from build123d import *

# Parameters (mm, degrees)
F0_W          = 44.958
F0_H          = 48.133
F1_DEPTH      = 0.8001
F2_R          = 5.207
F3_DEPTH      = 25.4
F3_DEPTH_BACK = 6.35
F4_W          = 12.7
F4_H          = 35.433
F5_DEPTH      = 19.05


with BuildPart() as f1:
    # F0 (on Top) → F1 (new body, symmetric)
    with BuildSketch(Plane.XY):
        Rectangle(F0_W, F0_H)
    extrude(amount=F1_DEPTH, both=True)



with BuildPart() as f3:
    # F2 (on face) → F3 (new body, two sides)
    with BuildSketch(Plane.XZ.offset(24.0665)) as f3_sk:
        with Locations((11.684, 11.5189)):
            Circle(F2_R)
    extrude(amount=F3_DEPTH)
    extrude(f3_sk.sketch, amount=-F3_DEPTH_BACK)


with BuildPart() as f1_1:
    add(f1.part)

    add(f3.part)  # F5 merges F3
    # F4 (on face) → F5 (join)
    with BuildSketch(Plane.XY.offset(0.8001)):
        with Locations((11.684, 0)):
            Rectangle(F4_W, F4_H)
    extrude(amount=F5_DEPTH)


solid = f1_1.part
Can you work these out from the model? Positions are in its coordinate system, mm. A direction names the side the tool comes from. Coordinates: 2 decimals unless noted, no trailing zeros. Loops run counter-clockwise (first coordinate to the right, second up) from the corner with the lowest first, then second, coordinate; pieces in that order, holes last. Notation, with made-up numbers: M 33,-5 L 74,-5 A17 cw 74,4 Z; hole C 61,58.25 d3. An arc over 180 degrees is marked long. Return JSON: item names as keys, results as strings. Group by question number.
Item 1: On a 3-axis mill with a long thin cutter (end or side, diameter ignored), from which of +Z, -Z, +X, -X, +Y, -Y can I reach the whole of each face in a straight line? I mean faces 1 (the flat face through (0, -24.066, 0)), 2 (the flat face through (18.034, 0, 10)), 3 (the flat face through (12, -17.716, 6)), 4 (the flat face through (12, 17.716, 10)). Say none if no direction works.
Item 2: Imagine slicing it at A-A (y = -16). Please give me the cut outline in (x, z), and give its area (3 significant figures).
Item 3: I'm going to push flat-ended pins straight in: pin 1 Ø5 at (x, z) = (12.5, 1.5) entering from +Y; pin 2 Ø1.5 at (y, z) = (-15.5, 7.5) entering from -X; pin 3 Ø1.5 at (y, z) = (-3, 4.5) entering from +X; pin 4 Ø4 at (y, z) = (-21, 7) entering from +X. Where does each tip first touch, or does it pass through?
Item 4: If I drill on L1, parallel to Z at x = -4, y = -22; L2, parallel to X at y = 9.5, z = 18.5; L3, parallel to Y at x = 18, z = 11.25, over which ranges is the centre line in solid material (lowest first)? Write a range as from..to.
Item 5: Imagine slicing it at B-B (z = 14.75). Please give me the cut outline in (x, y), and give its area (3 significant figures).
Item 6: Imagine slicing it at D-D (z = 1.75). Please give me the cut outline in (x, y).
Item 7: Imagine slicing it at C-C (x = 14.5). Please give me the cut outline in (y, z).
Verdict:
{
 "1": {"face 1": "-Z, +X, -X, -Y", "face 2": "+Z, +X, +Y, -Y", "face 3": "-Y", "face 4": "+Z, +X, -X, +Y"},
 "2": {"outline": "M -22.48,-0.8 L 22.48,-0.8 L 22.48,0.8 L 18.03,0.8 L 18.03,19.85 L 5.33,19.85 L 5.33,0.8 L -22.48,0.8 Z", "area": "314 mm^2"},
 "3": {"pin 1": "stops at y = 24.07", "pin 2": "stops at x = 5.33", "pin 3": "stops at x = 18.03", "pin 4": "stops at x = 16.24"},
 "4": {"L1": "z = -0.8..0.8", "L2": "x = 5.33..18.03", "L3": "y = -17.72..17.72"},
 "5": {"outline": "M 5.33,-17.72 L 7.6,-17.72 L 7.6,-49.47 L 15.77,-49.47 L 15.77,-17.72 L 18.03,-17.72 L 18.03,17.72 L 5.33,17.72 Z", "area": "709 mm^2"},
 "6": {"outline": "M 5.33,-17.72 L 18.03,-17.72 L 18.03,17.72 L 5.33,17.72 Z"},
 "7": {"outline": "M -49.47,7.14 L -17.72,7.14 L -17.72,0.8 L -24.07,0.8 L -24.07,-0.8 L 24.07,-0.8 L 24.07,0.8 L 17.72,0.8 L 17.72,19.85 L -17.72,19.85 L -17.72,15.9 L -49.47,15.9 Z"}
}
